```python
from build123d import *

# Parameters (mm, degrees)
SKETCH1_W           = 7
SKETCH1_H           = 7
SKETCH1_R           = 3
BOSS_EXTRUDE1_DEPTH = 12
CUT_EXTRUDE1_DEPTH  = 8
SKETCH5_W           = 17.899494936
SKETCH5_H           = 15
BOSS_EXTRUDE3_DEPTH = 2
SKETCH7_R           = 3
CUT_EXTRUDE3_DEPTH  = 17.242640687
CUT_EXTRUDE2_DEPTH  = 12
FILLET3_R           = 3


with BuildPart() as part:
    # Sketch1 → Boss-Extrude1 (new body)
    with BuildSketch(Plane.XY):
        Rectangle(SKETCH1_W, SKETCH1_H)
        Circle(SKETCH1_R, mode=Mode.SUBTRACT)
    extrude(amount=BOSS_EXTRUDE1_DEPTH)

    # Sketch3 → Cut-Extrude1 (cut, through all)
    with BuildSketch(Plane(origin=(0, 3.5, 0), x_dir=(1, 0, 0), z_dir=(0, 1, 0))):
        Polygon((-3.5, -12), (3.5, -12), (-3.5, -5), align=None)
    extrude(amount=-CUT_EXTRUDE1_DEPTH, mode=Mode.SUBTRACT)

    # Sketch5 → Boss-Extrude3 (add)
    with BuildSketch(Plane(origin=(-4.25, 0, 4.25), x_dir=(0.707106781, 0, 0.707106781), z_dir=(-0.707106781, 0, 0.707106781))):
        with Locations((6.01040764, 0)):
            Rectangle(SKETCH5_W, SKETCH5_H)
    extrude(amount=BOSS_EXTRUDE3_DEPTH)

    # Sketch7 → Cut-Extrude3 (cut, through all)
    with BuildSketch(Plane(origin=(0, 0, 0), x_dir=(-1, 0, 0), z_dir=(0, 0, -1))):
        Circle(SKETCH7_R)
    extrude(amount=-CUT_EXTRUDE3_DEPTH, mode=Mode.SUBTRACT)

    # Sketch6 → Cut-Extrude2 (cut, through all)
    with BuildSketch(Plane(origin=(0, 3.5, 0), x_dir=(1, 0, 0), z_dir=(0, 1, 0))):
        Polygon((-3.5, 0), (3.5, -7), (3.5, 0), align=None)
    extrude(amount=-CUT_EXTRUDE2_DEPTH, mode=Mode.SUBTRACT)

    # Fillet3
    fillet3_edges = [part.edges().sort_by_distance(p)[0] for p in [
        (5.621320344, -7.5, 15.535533906),
        (5.621320344, 7.5, 15.535533906),
        (-7.035533906, 7.5, 2.878679656),
        (-7.035533906, -7.5, 2.878679656),
    ]]
    fillet(fillet3_edges, radius=FILLET3_R)


solid = part.part
```
The model under review builds one solid part; all positions refer to its coordinate system, in mm. A direction names the side the tool comes from. Coordinates: 2 decimals unless noted, no trailing zeros. Write each loop counter-clockwise with the first axis right and the second up, starting at its lowest first coordinate (ties: lowest second). Pieces come first, ordered by that corner, then holes. Notation, with made-up numbers: (70, -13) - (84, -13) arc R7 ccw to (84, -8) - close; hole circle Ø8 at (7, 86.25). An arc over 180 degrees is marked (long way). Answer in a Markdown table with one row per item. Add a question column.
Q1. Consider section D-D on y = 5.5. Give the boundary of the cut face in (x, z).
Q2. Consider section B-B on x = 1.25. Give the boundary of the cut face in (y, z), then the cut area to 3 significant figures.
Q3. Consider section C-C on z = 11.25. Give the boundary of the cut face in (x, y).
Q4. To check wall thickness, follow line 1 along Y through (x, z) = (0, 8); line 2 along Y through (x, z) = (0, 8.75); line 3 along X through (y, z) = (0, 8). State the ranges of each line that lie inside material, in increasing order. Write a range as from..to.
Q5. Consider section A-A on y = 2. Give the boundary of the cut face in (x, z), then the cut area to 3 significant figures.
Q6. For faces 1 (the face through (0, -3.5, 6)), 2 (the face through (-6.441, 6.598, 3.493)), 3 (the face through (-7.026, -0.063, 2.869)), 4 (the face through (0, 3.5, 6)), 5 (the face through (3.5, 0, 9)), list the 3-axis set-ups (+Z, -Z, +X, -X, +Y, -Y) from which the entire face can be reached by the end or side of a thin tool; tool diameter is ignored.
Q7. Clearance check with flat-ended pins moving along their axes: pin 1 (3.5 mm diameter, centred on x = 0, z = 4.5, fed in from +Y); pin 2 (1.5 mm diameter, centred on y = 0, z = 10, fed in from +X); pin 3 (5.5 mm diameter, centred on x = 0, y = 0, fed in from +Z); pin 4 (1 mm diameter, centred on x = -4.5, y = -3, fed in from +Z). State where each tip first meets the part, or that it passes through.
Q8. Draft analysis for pull direction X (two halves, no side actions). For faces 6 (the face through (-6.441, -6.598, 3.493)), 7 (the face through (-1, -7.5, 9)), 8 (the face through (4.974, 6.645, 14.908)), 9 (the face through (-3.5, 0, 2)), state which applies: +X half, -X half, draft (parallel to the pull), parting line (faces both ways), or undercut.
Answers below:
| question | item | result |
|---|---|---|
| 1 | outline | (-7.62, 3.71) - (-6.21, 2.29) - (6.21, 14.71) - (4.79, 16.12) - close |
| 2 | outline | (-7.5, 9.75) - (-3.5, 9.75) - (-3.5, 4.75) - (-2.73, 4.75) - (-2.73, 12.58) - (-7.5, 12.58) - close; (2.73, 4.75) - (3.5, 4.75) - (3.5, 9.75) - (7.5, 9.75) - (7.5, 12.58) - (2.73, 12.58) - close |
| 2 | area | 34.7 mm² |
| 3 | outline | (-0.08, -7.5) - (2.75, -7.5) - (2.75, -3.5) - (3.5, -3.5) - (3.5, 3.5) - (2.75, 3.5) - (2.75, 7.5) - (-0.08, 7.5) - (-0.08, 3) arc R3 cw (long way) to (-0.08, -3) - close |
| 4 | line 1 | -3.5..-3, 3..3.5 |
| 4 | line 2 | -7.5..-3, 3..7.5 |
| 4 | line 3 | -3.33..-3, 3..3.5 |
| 5 | outline | (-7.74, 3.59) - (-6.33, 2.17) - (-3.5, 5) - (-3.5, 0) - (-2.24, 1.26) - (-2.24, 9.09) - close; (2.24, 5.74) - (3.5, 7) - (3.5, 12) - (6.33, 14.83) - (4.91, 16.24) - (2.24, 13.56) - close |
| 5 | area | 35.8 mm² |
| 6 | face 1 | -Z, +X, -Y |
| 6 | face 2 | -Z, -X, +Y |
| 6 | face 3 | -Z, -X, +Y, -Y |
| 6 | face 4 | -Z, +X, +Y |
| 6 | face 5 | -Z, +X, +Y, -Y |
| 7 | pin 1 | y = 3.5 |
| 7 | pin 2 | x = 3.5 |
| 7 | pin 3 | through |
| 7 | pin 4 | z = 7.33 |
| 8 | face 6 | -X half |
| 8 | face 7 | draft |
| 8 | face 8 | +X half |
| 8 | face 9 | undercut |
